from build123d import *

# Parameters (mm, degrees)
SKETCH1_R           = 25
BOSS_EXTRUDE1_DEPTH = 35
SKETCH2_R           = 17.5
CUT_EXTRUDE1_DEPTH  = 10
SKETCH7_W           = 90
SKETCH7_H           = 60
BOSS_EXTRUDE3_DEPTH = 15
SKETCH8_R           = 10
CUT_EXTRUDE4_DEPTH  = 40
CUT_EXTRUDE4_DRAFT  = 7
SKETCH9_W           = 10
SKETCH9_H           = 60
BOSS_EXTRUDE4_DEPTH = 30
SKETCH11_R          = 5
CUT_EXTRUDE5_DEPTH  = 35
SKETCH12_W          = 60
SKETCH12_H          = 15
BOSS_EXTRUDE5_DEPTH = 30
RIB1_START          = -6
RIB1_DEPTH          = 12
SKETCH16_R          = 6
CUT_EXTRUDE6_DEPTH  = 30
FILLET1_R           = 10
SKETCH17_R          = 7
CUT_EXTRUDE7_DEPTH  = 30


# Read off the part's stored shape, not the designer's step: Rib1
with BuildPart() as part:
    # Sketch1 → Boss-Extrude1 (new body)
    with BuildSketch(Plane(origin=(0, 0, 0), x_dir=(1, 0, 0), z_dir=(0, 1, 0))):
        with Locations(Location((0, 0, 0), (0, 0, 270))):
            Circle(SKETCH1_R)
    extrude(amount=BOSS_EXTRUDE1_DEPTH)

    # Sketch2 → Cut-Extrude1 (cut)
    with BuildSketch(Plane(origin=(0, 35, 0), x_dir=(1, 0, 0), z_dir=(0, 1, 0))):
        with Locations(Location((0, 0, 0), (0, 0, 270))):
            Circle(SKETCH2_R)
    extrude(amount=-CUT_EXTRUDE1_DEPTH, mode=Mode.SUBTRACT)

    # Sketch7 → Boss-Extrude3 (add)
    with BuildSketch(Plane.XZ):
        Rectangle(SKETCH7_W, SKETCH7_H)
    extrude(amount=BOSS_EXTRUDE3_DEPTH)


with BuildPart() as cut_extrude4_tool:
    # Sketch8 → Cut-Extrude4 (with draft: the straight prism first)
    with BuildSketch(Plane.XZ.offset(15)):
        Circle(SKETCH8_R)
    extrude(amount=-CUT_EXTRUDE4_DEPTH)
    # Cut-Extrude4: the draft: its side faces are tilted about the plane it starts from
    cut_extrude4_sides = [cut_extrude4_tool.faces().sort_by_distance(p)[0] for p in [
        (-10, 5, 0),
    ]]
    draft(cut_extrude4_sides, Plane.XZ.offset(15), CUT_EXTRUDE4_DRAFT)


with BuildPart() as part_1:
    add(part.part)

    # Cut-Extrude4: cut by cut_extrude4_tool
    add(cut_extrude4_tool.part, mode=Mode.SUBTRACT)

    # Sketch9 → Boss-Extrude4 (add)
    with BuildSketch(Plane.XZ.offset(15)):
        with Locations((-40, 0)):
            Rectangle(SKETCH9_W, SKETCH9_H)
        with Locations((40, 0)):
            Rectangle(SKETCH9_W, SKETCH9_H)
    extrude(amount=BOSS_EXTRUDE4_DEPTH)

    # Sketch11 → Cut-Extrude5 (cut, symmetric)
    with BuildSketch(Plane(origin=(0, 0, 0), x_dir=(0, 0, -1), z_dir=(1, 0, 0))):
        with Locations((0, 14)):
            Circle(SKETCH11_R)
    extrude(amount=CUT_EXTRUDE5_DEPTH, both=True, mode=Mode.SUBTRACT)

    # Sketch12 → Boss-Extrude5 (add)
    with BuildSketch(Plane(origin=(45, 0, 0), x_dir=(0, 0, -1), z_dir=(1, 0, 0))):
        with Locations((0, -37.5)):
            Rectangle(SKETCH12_W, SKETCH12_H)
    boss_extrude5 = extrude(amount=BOSS_EXTRUDE5_DEPTH)

    # Mirror1: Boss-Extrude5 across plane
    add(boss_extrude5.mirror(Plane(origin=(0, 0, 0), x_dir=(0, 0, 1), z_dir=(1, 0, 0))))

    # Rib1 outline → Rib1 (add)
    with BuildSketch(Plane.XY.offset(RIB1_START)):
        Polygon((-35, -15), (-35, -45), (-20, -15), align=None)
    rib1 = extrude(amount=RIB1_DEPTH)

    # Mirror2: Rib1 across plane
    add(rib1.mirror(Plane(origin=(0, 0, 0), x_dir=(0, 0, 1), z_dir=(1, 0, 0))))

    # Sketch16 → Cut-Extrude6 (cut)
    with BuildSketch(Plane(origin=(0, -30, 0), x_dir=(1, 0, 0), z_dir=(0, 1, 0))):
        with Locations(Location((-60, -15, 0), (0, 0, 270))):
            Circle(SKETCH16_R)
        with Locations(Location((-60, 15, 0), (0, 0, 90))):
            Circle(SKETCH16_R)
    extrude(amount=-CUT_EXTRUDE6_DEPTH, mode=Mode.SUBTRACT)

    # Fillet1
    fillet1_edges = [part_1.edges().sort_by_distance(p)[0] for p in [
        (-75, -37.5, 30),
        (-75, -37.5, -30),
    ]]
    fillet(fillet1_edges, radius=FILLET1_R)

    # Sketch17 → Cut-Extrude7 (cut)
    with BuildSketch(Plane(origin=(0, -30, 0), x_dir=(1, 0, 0), z_dir=(0, 1, 0))):
        with Locations((75, 0)):
            Circle(SKETCH17_R)
    extrude(amount=-CUT_EXTRUDE7_DEPTH, mode=Mode.SUBTRACT)


solid = part_1.part
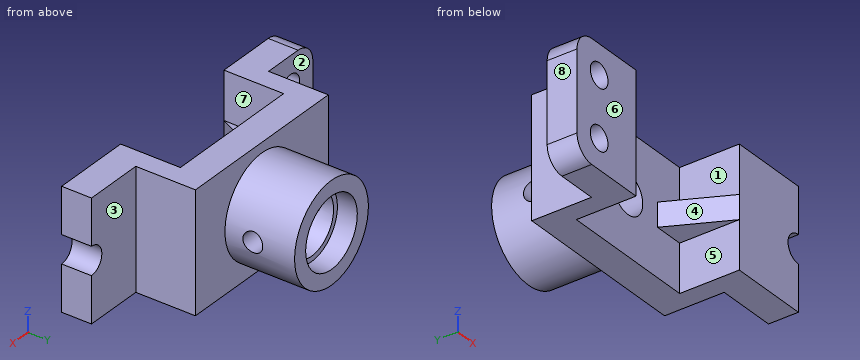
The listing builds one solid part. Answer for the finished solid, in the listing's coordinates (mm). Face numbers are marked on the shaded views. A direction names the side the tool comes from. Round coordinates to 2 decimals unless told otherwise and drop trailing zeros. Order: outer loops, then holes, each group sorted by start corner. A loop starts at its lowest first (then second) coordinate and runs counter-clockwise, first axis right, second up. Notation, with made-up numbers: (52, 59.5) -> (86, 59.5) arc R29 ccw to (86, 97.5) -> close; hole circle Ø11 at (59, 35). An arc over 180 degrees is marked (long way). One line per item, written item: value.
Item 1: Given P1, Ø15, axis at y = -16, z = 8, coming from the -X side; P2, Ø15, axis at x = -63.5, z = -10, coming from the +Y side; P3, Ø7, axis at x = -60, z = 15, coming from the +Y side; P4, Ø24, axis at y = -9.5, z = 2, coming from the +X side, each flat-ended and moving along its own axis, determine where each tip first touches the part or whether it passes through.
Taken from the geometry:
P1: stops at x = -45
P2: stops at y = -30
P3: passes through
P4: stops at x = 45
Item 2: For a pull along X with two mould halves and no side action, classify the marked faces 6, 7 and 8 as released by +X, released by -X, zero draft, split by the parting line, or undercut.
Taken from the geometry:
face 6: zero draft
face 7: undercut
face 8: released by -X
Item 3: For the marked faces 1, 2, 3, 4 and 5, determine the directions among +Z, -Z, +X, -X, +Y, -Y from which every point of the face is accessible in a straight line to the end or side of a thin tool.
Taken from the geometry:
face 1: +Z, -Y
face 2: +Z, -Z, -X, +Y
face 3: +Z, -Z, +X, +Y
face 4: +Z, -Z, -Y
face 5: -Z, -Y
Item 4: Find section B-B, the plane y = 14. Give the vertices of the cut face in (x, z).
Taken from the geometry:
outline: (-24.49, -5) arc R25 ccw to (24.49, -5) -> (12.61, -5) arc R13.56 cw to (-12.61, -5) -> close; (-24.49, 5) -> (-12.61, 5) arc R13.56 cw to (12.61, 5) -> (24.49, 5) arc R25 ccw to start
Item 5: Find section D-D, the plane x = -26.5. Give the vertices of the cut face in (y, z).
Taken from the geometry:
outline: (-28, -6) -> (-15, -6) -> (-15, -30) -> (0, -30) -> (0, 30) -> (-15, 30) -> (-15, 6) -> (-28, 6) -> close
Item 6: Find section A-A, the plane x = 0. Give the vertices of the cut face in (y, z).
Taken from the geometry:
outline: (-15, -30) -> (0, -30) -> (0, -25) -> (35, -25) -> (35, -17.5) -> (25, -17.5) -> (25, -14.91) -> (-15, -10) -> close; (-15, 10) -> (25, 14.91) -> (25, 17.5) -> (35, 17.5) -> (35, 25) -> (0, 25) -> (0, 30) -> (-15, 30) -> close
Item 7: Straight lines are drawn through the part: L1, parallel to X at y = -25, z = 25; L2, parallel to Z at x = -62.5, y = -34; L3, parallel to X at y = -34, z = 7.5. For each, find the intervals that lie inside material, in ascending order.
Taken from the geometry:
L1: x = -45 to -35, 35 to 45
L2: z = -30 to -20.45, -9.55 to 9.55, 20.45 to 30
L3: x = -75 to -35, 35 to 75
Item 8: Find section C-C, the plane z = 0. State how many separate pieces and enclosed holes the cut face has, then the cut area to 3 significant figures.
Taken from the geometry:
separate pieces: 4
enclosed holes: 0
area: 3,370 mm2
